Design review of the part shown in the three views and the two pictorial views. Dimensions are in mm from the part's minimum x, y and z. Coordinates: 2 decimals unless noted, no trailing zeros. Loops run counter-clockwise (first coordinate to the right, second up) from the corner with the lowest first, then second, coordinate; pieces in that order, holes last. Notation, with made-up numbers: (78.25, 11) -> (108.25, 11) arc R20 cw to (108.25, 22) -> close; hole circle Ø1 at (-10, -34). An arc over 180 degrees is marked (long way). One line per item, written item: value. Start each with the question number.
1. Add section D-D on x = 30. Write out the cut boundary in (y, z), plus the area to 3 significant figures.
2. Insertion check: pin 1 (3.5 mm diameter, centred on x = 37, z = 12, fed in from +Y); pin 2 (1.2 mm diameter, centred on x = 37.5, z = 11.5, fed in from +Y). Each pin has a flat end and moves straight along its axis. Give the tip position at first contact, or say it passes through.
3. Add section C-C on y = 1.45. Write out the cut boundary in (x, z).
4. Add section B-B on x = 50. Write out the cut boundary in (y, z).
5. Add section A-A on z = 12. Write out the cut boundary in (x, y), plus the area to 3 significant figures.
6. For probe 1 along X at (y, z) = (0.9, 12); probe 2 along X at (y, z) = (4.3, 12); probe 3 along Z at (x, y) = (37, 3.95), list the stretches that pass through material, from the lowest coordinate up.
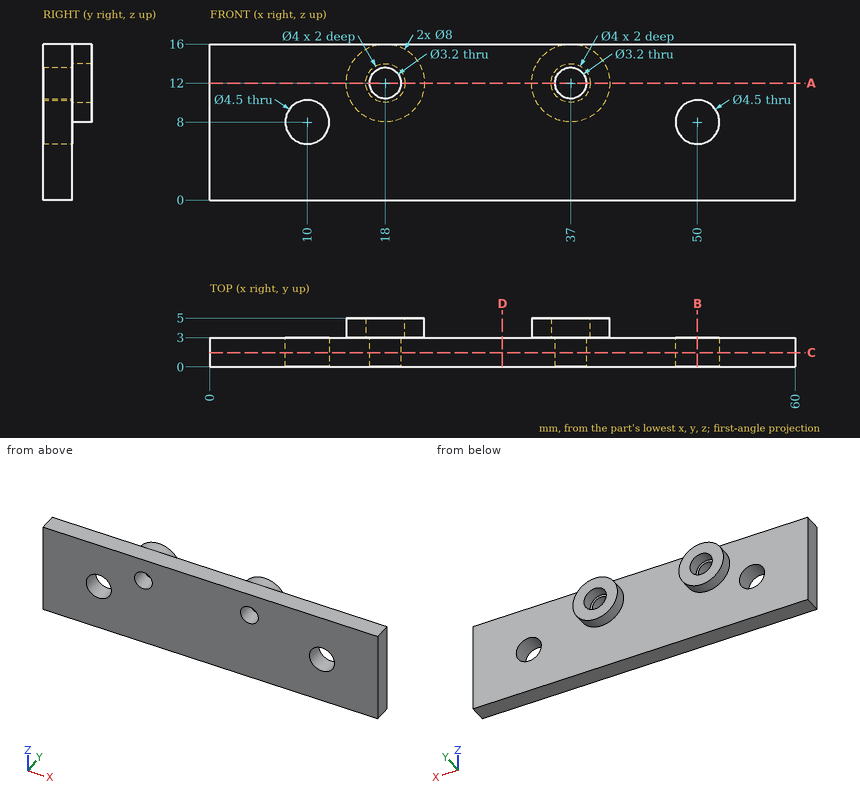
Worked answers:
1. outline: (0, 0) -> (3, 0) -> (3, 16) -> (0, 16) -> close
1. area: 48.0 mm²
2. pin 1: stops at y = 3
2. pin 2: passes through
3. outline: (0, 0) -> (60, 0) -> (60, 16) -> (0, 16) -> close; hole circle Ø4.5 at (10, 8); hole circle Ø3.2 at (18, 12); hole circle Ø3.2 at (37, 12); hole circle Ø4.5 at (50, 8)
4. outline: (0, 0) -> (3, 0) -> (3, 5.75) -> (0, 5.75) -> close; (0, 10.25) -> (3, 10.25) -> (3, 16) -> (0, 16) -> close
5. outline: (0, 0) -> (16.4, 0) -> (16.4, 3) -> (16, 3) -> (16, 5) -> (14, 5) -> (14, 3) -> (0, 3) -> close; (19.6, 0) -> (35.4, 0) -> (35.4, 3) -> (35, 3) -> (35, 5) -> (33, 5) -> (33, 3) -> (22, 3) -> (22, 5) -> (20, 5) -> (20, 3) -> (19.6, 3) -> close; (38.6, 0) -> (60, 0) -> (60, 3) -> (41, 3) -> (41, 5) -> (39, 5) -> (39, 3) -> (38.6, 3) -> close
5. area: 177 mm²
6. probe 1: x = 0 to 16.4, 19.6 to 35.4, 38.6 to 60
6. probe 2: x = 14 to 16, 20 to 22, 33 to 35, 39 to 41
6. probe 3: z = 8 to 10, 14 to 16
